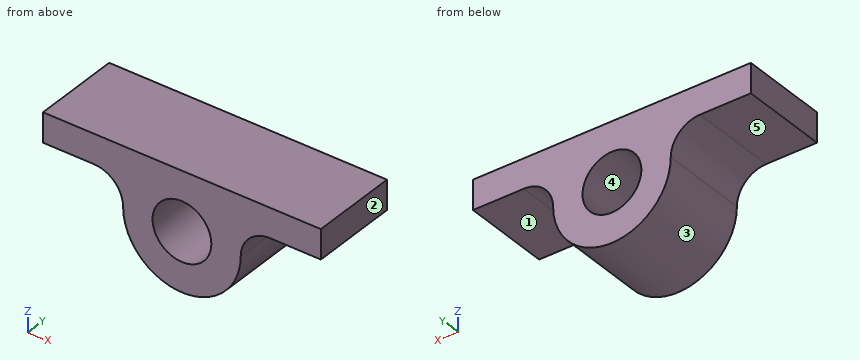
from build123d import *

# Parameters (mm, degrees)
SKETCH1_R           = 12.7
BOSS_EXTRUDE1_DEPTH = 38.1


with BuildPart() as part:
    # Sketch1 → Boss-Extrude1 (new body)
    with BuildSketch(Plane(origin=(0, 0, 0), x_dir=(1, 0, 0), z_dir=(0, 1, 0))):
        with BuildLine():
            ThreePointArc((25.4, 0), (29.119743879, -8.980256121), (38.1, -12.7))
            Line((38.1, -12.7), (60, -12.7))
            Line((60, -12.7), (60, -25.4))
            Line((60, -25.4), (-60, -25.4))
            Line((-60, -25.4), (-60, -12.7))
            Line((-60, -12.7), (-38.1, -12.7))
            ThreePointArc((-38.1, -12.7), (-29.119743879, -8.980256121), (-25.4, 0))
            ThreePointArc((-25.4, 0), (0, 25.4), (25.4, 0))
        make_face()
        Circle(SKETCH1_R, mode=Mode.SUBTRACT)
    extrude(amount=BOSS_EXTRUDE1_DEPTH)


solid = part.part
Input: part model. Units: mm. Frame: model coordinates. Face numbers are marked on the shaded views. A direction names the side the tool comes from. Round coordinates to 2 decimals unless told otherwise and drop trailing zeros. Order: outer loops, then holes, each group sorted by start corner. A loop starts at its lowest first (then second) coordinate and runs counter-clockwise, first axis right, second up. Notation, with made-up numbers: (86, 5) - (132, 5) arc R19 ccw to (132, 23) - close; hole circle Ø4 at (65.5, 49.25). An arc over 180 degrees is marked (long way). Answer as a JSON object with one key per item and string values. Group by question number.
(1) Cut plane C-C (z = -3.5). Return loops of the section in (x, y), then the cut area to 3 significant figures.
(2) Reachability of the marked faces 1 and 2 from +Z, -Z, +X, -X, +Y, -Y: full face, straight path, thin tool, end or side. Return the list, or none.
(3) Cut plane B-B (y = 10). Return loops of the section in (x, z).
(4) Material intervals for probe 1 along Z at (x, y) = (0, 29); probe 2 along X at (y, z) = (7.5, -0.5); probe 3 along X at (y, z) = (3, -8.5), sorted ascending. Write a range as from..to.
(5) Cut plane A-A (x = 0). Return loops of the section in (y, z).
(6) Draft query along X for the marked faces 3, 4 and 5. Return one class per face: released by +X, released by -X, zero draft, split by the parting line, or undercut.
(7) Cut plane D-D (x = -51). Return loops of the section in (y, z).
(8) Pin query (flat end, axial travel): P1, Ø17.5, axis at x = -49, y = 16.5, coming from the -Z side; P2, Ø4, axis at x = 9, y = 10.5, coming from the -Z side; P3, Ø8, axis at x = -27.5, y = 6, coming from the -Z side; P4, Ø4, axis at x = 37, z = 10, coming from the -Y side. Return the tip coordinate at first contact, or that it passes through.
Here are the results:
{
 "1": {"outline": "(-25.16, 0) - (-12.21, 0) - (-12.21, 38.1) - (-25.16, 38.1) - close; (12.21, 0) - (25.16, 0) - (25.16, 38.1) - (12.21, 38.1) - close", "area": "987 mm^2"},
 "2": {"face 1": "-Z, +X, +Y, -Y", "face 2": "+Z, -Z, +X, +Y, -Y"},
 "3": {"outline": "(-60, 12.7) - (-38.1, 12.7) arc R12.7 cw to (-25.4, 0) arc R25.4 ccw to (25.4, 0) arc R12.7 cw to (38.1, 12.7) - (60, 12.7) - (60, 25.4) - (-60, 25.4) - close; hole circle Ø25.4 at (0, 0)"},
 "4": {"probe 1": "z = -25.4..-12.7, 12.7..25.4", "probe 2": "x = -25.4..-12.69, 12.69..25.4", "probe 3": "x = -23.94..-9.44, 9.44..23.94"},
 "5": {"outline": "(0, -25.4) - (38.1, -25.4) - (38.1, -12.7) - (0, -12.7) - close; (0, 12.7) - (38.1, 12.7) - (38.1, 25.4) - (0, 25.4) - close"},
 "6": {"face 3": "split by the parting line", "face 4": "undercut", "face 5": "zero draft"},
 "7": {"outline": "(0, 12.7) - (38.1, 12.7) - (38.1, 25.4) - (0, 25.4) - close"},
 "8": {"P1": "stops at z = 12.7", "P2": "stops at z = -24.42", "P3": "stops at z = -9.64", "P4": "passes through"}
}
